Autodesk Inventor part; units mm, degrees
ref_plane "Work Plane1" through (-4.5, -2.1794, 0) normal (-1, 0, 0) x (0, 0, 1)
ref_plane "Work Plane2" through (4.5, -2.1794, 0) normal (1, 0, 0) x (0, 0, -1)
ref_plane "YZ Plane" through (0, 0, 0) normal (1, 0, 0) x (0, 1, 0)
sketch "Sketch1" plane through (0, 0, 0) normal (0, 0, 1) x (1, 0, 0)
  line L0 (-4.5, 0) -> (4.5, 0) construction
  line L1 (0, 7.6) -> (0, -7.6) construction
  line L2 (0, 7.6) -> (-1.6, 7.6)
  line L3 (-1.6, 7.6) -> (-4.5, 2.1794)
  line L4 (-4.5, 2.1794) -> (-4.5, 0)
  arc A0 (0, 5) -> (-4.5, 2.1794) centre (0, 0) ccw construction
  line L5 (0, 7.6) -> (1.6, 7.6)
  line L6 (1.6, 7.6) -> (4.5, 2.1794)
  line L7 (4.5, 2.1794) -> (4.5, 0)
  line L8 (0, -7.6) -> (-1.6, -7.6)
  line L9 (-1.6, -7.6) -> (-4.5, -2.1794)
  line L10 (-4.5, -2.1794) -> (-4.5, 0)
  line L11 (0, -7.6) -> (1.6, -7.6)
  line L12 (1.6, -7.6) -> (4.5, -2.1794)
  line L13 (4.5, -2.1794) -> (4.5, 0)
  point P0 (0, -5)
  dimension "d0" = 3.2
  dimension "d1" = 15.2
  dimension "d2" = 9
  dimension "d3" = 10
extrude "Extrusion1" add sketch "Sketch1" along normal blind 2
sketch "Sketch2" plane through (0, 0, 0) normal (0, 0, 1) x (1, 0, 0)
  circle A0 centre (0, 5.7) radius 1
  circle A1 centre (0, -5.7) radius 1
  line L0 (-6.3, 0) -> (6.3, 0)
  point P0 (0, 0)
  dimension "d6" = 2
  dimension "d7" = 11.4
extrude "Extrusion2" cut sketch "Sketch2" along normal through all
sketch "Sketch3" plane through (0, 0, 0) normal (1, 0, 0) x (0, 1, 0)
  line L0 (-6.7, 2) -> (-4.7, 2)
  line L1 (-4.7, 2) -> (-4.2, 3.8)
  line L2 (-4.2, 3.8) -> (0, 5.8)
  line L3 (0, 5.8) -> (4.2, 3.8) construction
  line L4 (4.7, 2) -> (6.7, 2)
  line L5 (4.2, 3.8) -> (4.7, 2) construction
  line L6 (0, 5.8) -> (0, 2)
  line L7 (2.1794, 2) -> (-2.1794, 2)
  line L8 (0, 2) -> (-4.7, 2)
  point P0 (0, 0)
  dimension "d10" = 5.8
  dimension "d11" = 3.8
  dimension "d12" = 8.4
revolve "Revolution1" add sketch "Sketch3" angle 360 about axis through (0, 0, 5.8) along (0, 0, -1)
sketch "Sketch4" plane through (0, 0, 2) normal (0, 0, 1) x (1, 0, 0)
  circle A0 centre (0, -5.7) radius 1
  circle A1 centre (0, -5.7) radius 1.5
  circle A2 centre (0, 5.7) radius 1
  circle A3 centre (0, 5.7) radius 1.5
  point P0 (0, 4.7)
  dimension "d14" = 3
extrude "Extrusion3" cut sketch "Sketch4" along normal through all contours A0 | A1 | A2 | A3
sketch "Sketch5" plane through (0, 0, 0) normal (0, 0, -1) x (-1, 0, 0)
  circle A0 centre (0, 0) radius 3.5
  circle A1 centre (0, 0) radius 2.7
  dimension "d17" = 7
  dimension "d18" = 5.4
extrude "Extrusion4" add sketch "Sketch5" along normal blind 0.8
ref_plane "Work Plane1" through (-4.5, -2.1794, 0) normal (-1, 0, 0) x (0, 0, 1)
split "Split1" plane through (-4.5, -2.1794, 0) removes the side toward (-1, 0, 0)
ref_plane "Work Plane2" through (4.5, -2.1794, 0) normal (1, 0, 0) x (0, 0, -1)
split "Split2" plane through (4.5, -2.1794, 0) removes the side toward (1, 0, 0)
properties part number "b10"
The model under review builds one solid part; all positions refer to its coordinate system, in mm. A direction names the side the tool comes from. Round coordinates to 2 decimals unless told otherwise and drop trailing zeros. Loops run counter-clockwise (first coordinate to the right, second up) from the corner with the lowest first, then second, coordinate; pieces in that order, holes last. Notation, with made-up numbers: (47, 88.25) -> (57, 88.25) arc R34 ccw to (57, 125.25) -> close; hole circle Ø6 at (-3, 18). An arc over 180 degrees is marked (long way). Return JSON: item names as keys, results as strings.
(1) Add section A-A on z = 0.75. Write out the cut boundary in (x, y).
Solved:
{"outline": "(-4.5, -2.18) -> (-1.6, -7.6) -> (1.6, -7.6) -> (4.5, -2.18) -> (4.5, 2.18) -> (1.6, 7.6) -> (-1.6, 7.6) -> (-4.5, 2.18) -> close; hole circle Ø2 at (0, -5.7); hole circle Ø2 at (0, 5.7)"}
(2) For faces 1 (the cylindrical face through (0, 4.2, 2.7)), 2 (the flat face through (0, 0, 0)), 3 (the cylindrical face through (0, -4.2, 2.7)), list the 3-axis set-ups (+Z, -Z, +X, -X, +Y, -Y) from which the entire face can be reached by the end or side of a thin tool; tool diameter is ignored.
Solved:
{"face 1": "+Z, +Y", "face 2": "-Z", "face 3": "+Z, -Y"}
(3) Add section C-C on x = -0.75. State how many separate pieces and enclosed holes the cut face has, plus the area to 3 significant figures.
Solved:
{"separate pieces": "3", "enclosed holes": "0", "area": "49.6 mm2"}
(4) Add section B-B on y = -6. Write out the cut boundary in (x, z).
Solved:
{"outline": "(-2.46, 0) -> (-0.95, 0) -> (-0.95, 2) -> (-2.46, 2) -> close; (0.95, 0) -> (2.46, 0) -> (2.46, 2) -> (0.95, 2) -> close"}
(5) For line 1 (Y direction, x = 0, z = 0.85); line 2 (Y direction, x = 0, z = -0.3); line 3 (Z direction, x = -1.25, y = -6.75), list the stretches that pass through material, from the lowest coordinate up.
Solved:
{"line 1": "-7.6 to -6.7, -4.7 to 4.7, 6.7 to 7.6", "line 2": "-3.5 to -2.7, 2.7 to 3.5", "line 3": "0 to 2"}
(6) For pin 1 (5 mm diameter, centred on x = -0.5, y = 3.5, fed in from +Z); pin 2 (3 mm diameter, centred on x = 2.5, z = 3, fed in from +Y); pin 3 (2 mm diameter, centred on y = 4, z = 0, fed in from +X); pin 4 (2.5 mm diameter, centred on x = 0, y = -5.7, fed in from +Z), all flat-tipped, find the tip position at first contact; note any pin that passes through.
Solved:
{"pin 1": "z = 5.31", "pin 2": "y = 7.6", "pin 3": "x = 4.06", "pin 4": "z = 2"}
(7) The part is to be moulded in two halves that separate along Y. For faces 4 (the flat face through (-1, 5, 2)), 5 (the flat face through (3.03, -4.93, 0.99)), 6 (the cylindrical face through (-0.217, -4.724, 0.986)), say which applies: released by +Y, released by -Y, zero draft, split by the parting line, or undercut.
Solved:
{"face 4": "zero draft", "face 5": "released by -Y", "face 6": "undercut"}
(8) Add section D-D on y = 5.7. Write out the cut boundary in (x, z).
Solved:
{"outline": "(-2.62, 0) -> (-1, 0) -> (-1, 2) -> (-2.62, 2) -> close; (1, 0) -> (2.62, 0) -> (2.62, 2) -> (1, 2) -> close"}
